```python
from build123d import *

# Parameters (mm, degrees)
F0_R      = 12.319
F0_R_2    = 11.938
F0_R_3    = 7.14375
F1_DEPTH  = 11.938
F0_R_4    = 17.018
F2_DEPTH  = 7.62
F0_R_5    = 27.305
F0_R_6    = 22.987
F3_DEPTH  = 4.699
F4_SIZE   = 1.524
F5_SIZE   = 0.762
F6_R      = 1.4732
F6_R_2    = 1.7907
F7_DEPTH  = 25.4
F8_DEPTH  = 2.286
F9_R      = 1.0922
F10_DEPTH = 9.652


with BuildPart() as f1:
    # F0 (on Right) → F1 (new body)
    with BuildSketch(Plane.YZ):
        Circle(F0_R)
        Circle(F0_R_2, mode=Mode.SUBTRACT)
        Circle(F0_R_2)
        Circle(F0_R_3, mode=Mode.SUBTRACT)
    extrude(amount=-F1_DEPTH)

    # F0 (on Right) → F2 (join)
    with BuildSketch(Plane.YZ):
        Circle(F0_R_4)
        Circle(F0_R, mode=Mode.SUBTRACT)
    extrude(amount=-F2_DEPTH)

    # F0 (on Right) → F3 (join)
    with BuildSketch(Plane.YZ):
        Circle(F0_R_5)
        Circle(F0_R_6, mode=Mode.SUBTRACT)
        Circle(F0_R_6)
        Circle(F0_R_4, mode=Mode.SUBTRACT)
    extrude(amount=-F3_DEPTH)

    # F4
    f4_edges = [f1.edges().sort_by_distance(p)[0] for p in [
        (-11.938, -12.319, 0),
    ]]
    chamfer(f4_edges, length=F4_SIZE)

    # F5
    f5_edges = [f1.edges().sort_by_distance(p)[0] for p in [
        (-11.938, -7.14375, 0),
        (0, -7.14375, 0),
    ]]
    chamfer(f5_edges, length=F5_SIZE)

    # F6 (on face) → F7 (cut)
    with BuildSketch(Plane.YZ):
        with Locations((-12.573, 21.7678)):
            Circle(F6_R)
        with Locations((-21.7678, 12.573)):
            Circle(F6_R)
        with Locations((-21.7678, -12.573)):
            Circle(F6_R)
        with Locations((12.573, 21.7678)):
            Circle(F6_R)
        with Locations((21.7678, 12.573)):
            Circle(F6_R)
        with Locations((21.7678, -12.573)):
            Circle(F6_R)
        with Locations((12.573, -21.7678)):
            Circle(F6_R)
        with Locations((-12.573, -21.7678)):
            Circle(F6_R)
        with Locations((-14.3764, 14.3764)):
            Circle(F6_R_2)
        with Locations((14.3764, 14.3764)):
            Circle(F6_R_2)
        with Locations((14.3764, -14.3764)):
            Circle(F6_R_2)
        with Locations((-14.3764, -14.3764)):
            Circle(F6_R_2)
    extrude(amount=-F7_DEPTH, mode=Mode.SUBTRACT)

    # F0 (on Right) → F8 (cut)
    with BuildSketch(Plane.YZ):
        Circle(F0_R_6)
        Circle(F0_R_4, mode=Mode.SUBTRACT)
        Circle(F0_R_4)
        Circle(F0_R, mode=Mode.SUBTRACT)
        Circle(F0_R)
        Circle(F0_R_2, mode=Mode.SUBTRACT)
    extrude(amount=-F8_DEPTH, mode=Mode.SUBTRACT)

    # F9 (on face) → F10 (cut)
    with BuildSketch(Plane.YZ):
        with Locations((-8.128, 4.699)):
            Circle(F9_R)
        with Locations((0, 9.398)):
            Circle(F9_R)
        with Locations((8.128, 4.699)):
            Circle(F9_R)
        with Locations((8.128, -4.699)):
            Circle(F9_R)
        with Locations((0, -9.398)):
            Circle(F9_R)
        with Locations((-8.128, -4.699)):
            Circle(F9_R)
    extrude(amount=-F10_DEPTH, mode=Mode.SUBTRACT)


solid = f1.part
```
CAD build for the part. Positions are in the model's coordinates, mm. A direction names the side the tool comes from. Round coordinates to 2 decimals unless told otherwise and drop trailing zeros. Order: outer loops, then holes, each group sorted by start corner. A loop starts at its lowest first (then second) coordinate and runs counter-clockwise, first axis right, second up. Notation, with made-up numbers: (19.5, -40) -> (34.5, -40) arc R15 cw to (34.5, -30) -> close; hole circle Ø10 at (-14, -5.75). An arc over 180 degrees is marked (long way). Write item = value, one per line.
(1) Cut at C-C (y = 18). Write the cut outline in (x, z), plus the area to 3 significant figures.
Answers follow:
outline = (-4.7, -20.53) -> (0, -20.53) -> (0, -14.3) -> (-2.29, -14.3) -> (-2.29, 14.3) -> (0, 14.3) -> (0, 20.53) -> (-4.7, 20.53) -> close
area = 128 mm²
(2) Flat gauge pins, fed straight in: P1, Ø4.5, axis at y = 14.38, z = -14.38, coming from the +X side; P2, Ø4, axis at y = 12.57, z = -21.77, coming from the -X side; P3, Ø12, axis at y = -8.5, z = -20, coming from the -X side. Where does each tip first touch, or does it go through?
Answers follow:
P1 = -2.29
P2 = -4.7
P3 = -7.62
(3) Cut at B-B (x = -6.5). Write the cut outline in (y, z), plus the area to 3 significant figures.
Answers follow:
outline = circle Ø34.04 at (0, 0); hole circle Ø2.18 at (-8.13, -4.7); hole circle Ø2.18 at (-8.13, 4.7); hole circle Ø14.29 at (0, 0); hole circle Ø2.18 at (0, -9.4); hole circle Ø2.18 at (0, 9.4); hole circle Ø2.18 at (8.13, -4.7); hole circle Ø2.18 at (8.13, 4.7)
area = 727 mm²
(4) 3-axis set-ups, long thin cutter, end or side, ignore diameter. For faces 4 (the flat face through (-9.652, 0, 9)), 5 (the flat face through (-11.938, -6, 6)), 6 (the cylindrical face through (-8.997, -2.671, -12.026)): which of +Z, -Z, +X, -X, +Y, -Y reach the whole face in a straight line?
Answers follow:
face_4 = +X
face_5 = +Z, -Z, -X, +Y, -Y
face_6 = -X
(5) Pull direction Y, two halves, no side cores. Call faces 1 (the cylindrical face through (-2.317, -3.555, 27.073)), 2 (the flat face through (-9.652, 0, -9)), 3 (the flat face through (-4.699, 12, 13)): +Y half, -Y half, draft (parallel to the pull), parting line (faces both ways), or undercut.
Answers follow:
face_1 = parting line
face_2 = undercut
face_3 = draft
(6) Drill centre lines: L1, parallel to Z at x = -1.5, y = 8; L2, parallel to X at y = -2.5, z = -12; L3, parallel to Y at x = -2.25, z = -19. Where is each one in solid material? Low to high.
Answers follow:
L1 = -26.11 to -21.55, -8.86 to -5.78, -3.61 to 3.61, 5.78 to 8.86, 21.55 to 26.11
L2 = -10.48 to -2.29
L3 = -19.61 to -12.94, 12.94 to 19.61
(7) Cut at D-D (x = -3.25). State how many separate pieces and enclosed holes the cut face has, plus the area to 3 significant figures.
Answers follow:
separate_pieces = 1
enclosed_holes = 19
area = 2,060 mm²
